Model file for the job. Use its own axes, mm. Face numbers are marked on the shaded views. Round coordinates to 2 decimals unless told otherwise and drop trailing zeros. Loops run counter-clockwise (first coordinate to the right, second up) from the corner with the lowest first, then second, coordinate; pieces in that order, holes last. Notation, with made-up numbers: (49, -24.75) - (94, -24.75) arc R27 cw to (94, -8.75) - close; hole circle Ø5 at (-32, 6.25). An arc over 180 degrees is marked (long way). Use one line per item in the form item = value.
Autodesk Inventor part; units mm, degrees
ref_plane "YZ Plane" through (0, 0, 0) normal (1, 0, 0) x (0, 1, 0)
ref_plane "XZ Plane" through (0, 0, 0) normal (0, 1, 0) x (-1, 0, 0)
ref_plane "XY Plane" through (0, 0, 0) normal (0, 0, 1) x (1, 0, 0)
sketch "Sketch1" plane through (0, 0, 0) normal (0, 1, 0) x (-1, 0, 0)
  circle A0 centre (0, 0) radius 24.5
  circle A1 centre (0, 0) radius 22
  dimension "d0" = 49
  dimension "d1" = 44
extrude "Extrusion1" add sketch "Sketch1" along normal blind 0.5
sketch "Sketch2" plane through (0, 0.5, 0) normal (0, 1, 0) x (1, 0, 0)
  circle A0 centre (0, 0) radius 26.25
  dimension "d4" = 52.5
extrude "Extrusion2" add sketch "Sketch2" along normal blind 4
sketch "Sketch3" plane through (0, 0.5, 0) normal (0, -1, 0) x (1, 0, 0)
  circle A0 centre (0, 0) radius 17.5
  dimension "d7" = 35
extrude "Extrusion3" cut sketch "Sketch3" against normal blind 2.5
sketch "Sketch4" plane through (0, 3, 0) normal (0, -1, 0) x (1, 0, 0)
  circle A0 centre (0, 0) radius 11
  dimension "d10" = 22
extrude "Extrusion4" cut sketch "Sketch4" against normal blind 4
sketch "Sketch5" plane through (0, 3, 0) normal (0, -1, 0) x (1, 0, 0)
  circle A0 centre (0, 0) radius 11
  circle A1 centre (0, 0) radius 11
  circle A2 centre (0, 0) radius 12.5
  dimension "d13" = 25
extrude "Extrusion5" add sketch "Sketch5" along normal blind 1
sketch "Sketch6" plane through (0, 0.5, 0) normal (0, -1, 0) x (1, 0, 0)
  circle A0 centre (0, 0) radius 17.5
  circle A1 centre (0, 0) radius 22
  circle A2 centre (0, 0) radius 22
extrude "Extrusion6" cut sketch "Sketch6" against normal blind 2
sketch "Sketch7" plane through (0, 2.5, 0) normal (0, -1, 0) x (1, 0, 0)
  circle A0 centre (0, 0) radius 17.5
  circle A1 centre (0, 0) radius 18.5
  dimension "d18" = 37
extrude "Extrusion7" add sketch "Sketch7" along normal blind 1
chamfer "Chamfer1" distance 2 angle 45 1 edges at (-26.25, 4.5, 0)
properties part number "Grease retainer disk"
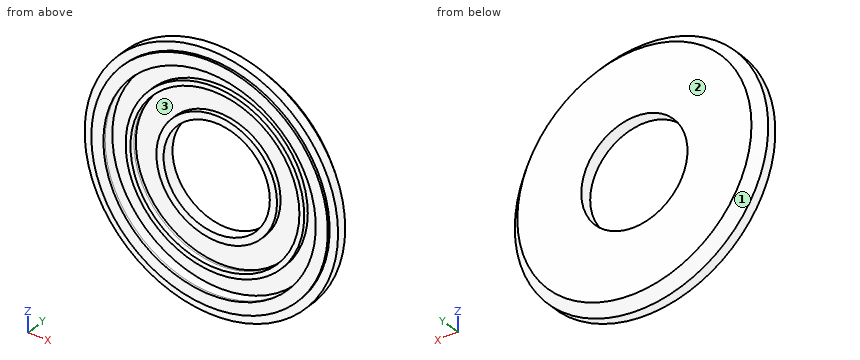
1. Wall check: probe 1 along Z at (x, y) = (0, 2.15); probe 2 along Z at (x, y) = (0, 0.3); probe 3 along Z at (x, y) = (0, 2.85). Give the ranges that are in metal, low to high.
Geometry check:
probe_1 = -26.25 to -22, -18.5 to -17.5, -12.5 to -11, 11 to 12.5, 17.5 to 18.5, 22 to 26.25
probe_2 = -24.5 to -22, 22 to 24.5
probe_3 = -25.9 to -17.5, -12.5 to -11, 11 to 12.5, 17.5 to 25.9
2. Flat gauge pins, fed straight in: pin 1 (10.5 mm diameter, centred on x = 0.5, z = 3.5, fed in from -Y); pin 2 (10 mm diameter, centred on x = 7.5, z = -15, fed in from -Y); pin 3 (13 mm diameter, centred on x = 4.5, z = 5.5, fed in from -Y); pin 4 (1 mm diameter, centred on x = -19, z = -6.5, fed in from -Y). Where does each tip first touch, or does it go through?
Geometry check:
pin_1 = through
pin_2 = 1.5
pin_3 = 2
pin_4 = 2.5
3. Cut at C-C, the plane y = 3.6. Give the cut face in (x, z), plus the area to 3 significant figures.
Geometry check:
outline = circle Ø50.3 at (0, 0); hole circle Ø22 at (0, 0)
area = 1,610 mm^2
4. Pull direction Z, two halves, no side cores. Call the marked faces 1, 2 and 3: +Z half, -Z half, draft (parallel to the pull), parting line (faces both ways), or undercut.
Geometry check:
face_1 = parting line
face_2 = draft
face_3 = undercut
